Check sheet for the modelled part. Datum: model origin and axes. Units: mm. Face numbers are marked on the shaded views. A direction names the side the tool comes from. Give positions to 0.01 mm unless a question says otherwise; leave off trailing zeros. Write each loop counter-clockwise with the first axis right and the second up, starting at its lowest first coordinate (ties: lowest second). Pieces come first, ordered by that corner, then holes. Notation, with made-up numbers: M -7.5,29 L 39.5,29 A22 ccw 39.5,47 Z; hole C 0.5,64.25 d2. An arc over 180 degrees is marked long. Write each question's results on one line, items separated by ' | '. Start each with the question number.
from build123d import *

# Parameters (mm, degrees)
SKETCH1_W                                  = 47
SKETCH1_H                                  = 47
BOSS_EXTRUDE1_DEPTH                        = 32
SKETCH2_W                                  = 44
SKETCH2_H                                  = 44
CUT_EXTRUDE1_DEPTH                         = 26.1
SKETCH3_W                                  = 3.5
SKETCH3_H                                  = 3.5
BOSS_EXTRUDE2_DEPTH                        = 20.5
MIRROR1_AT_THE_SECOND_PLANE_COPY_1_SKETC_W = 3.5
MIRROR1_AT_THE_SECOND_PLANE_COPY_1_SKETC_H = 3.5
MIRROR1_AT_THE_SECOND_PLANE_COPY_1_DEPTH   = 20.5
CUT_EXTRUDE3_REACH                         = 63.524
SKETCH4_W                                  = 2
SKETCH4_H                                  = 20
LPATTERN1_COUNT                            = 7
LPATTERN1_PITCH                            = 4
BOSS_EXTRUDE4_START                        = -1.5
SKETCH8_W                                  = 26
SKETCH8_H                                  = 2
BOSS_EXTRUDE4_DEPTH                        = 1.5
LPATTERN2_COUNT                            = 5
LPATTERN2_PITCH                            = 4
SKETCH6_W                                  = 47
SKETCH6_H                                  = 47
SKETCH6_W_2                                = 44
SKETCH6_H_2                                = 44
BOSS_EXTRUDE5_DEPTH                        = 3
SKETCH7_R                                  = 5
CUT_EXTRUDE4_DEPTH                         = 10
SKETCH10_W                                 = 10
SKETCH10_H                                 = 5
CUT_EXTRUDE5_DEPTH                         = 62.524385409
SKETCH12_W                                 = 12.571328749
SKETCH12_H                                 = 5
CUT_EXTRUDE6_DEPTH                         = 10


with BuildPart() as part:
    # Sketch1 → Boss-Extrude1 (new body)
    with BuildSketch(Plane(origin=(0, 0, 0), x_dir=(1, 0, 0), z_dir=(0, 1, 0))):
        Rectangle(SKETCH1_W, SKETCH1_H)
    extrude(amount=BOSS_EXTRUDE1_DEPTH)

    # Sketch2 → Cut-Extrude1 (cut)
    with BuildSketch(Plane.XZ):
        Rectangle(SKETCH2_W, SKETCH2_H)
    extrude(amount=-CUT_EXTRUDE1_DEPTH, mode=Mode.SUBTRACT)

    # Sketch3 → Boss-Extrude2 (add)
    with BuildSketch(Plane.XZ.offset(-26.1)):
        with Locations((-20.25, 20.25)):
            Rectangle(SKETCH3_W, SKETCH3_H)
    boss_extrude2 = extrude(amount=BOSS_EXTRUDE2_DEPTH)

    # Mirror1: Boss-Extrude2 across plane
    add(boss_extrude2.mirror(Plane(origin=(0, 0, 0), x_dir=(0, 0, 1), z_dir=(1, 0, 0))))

    # Mirror1 at the second plane: Boss-Extrude2 across plane
    add(boss_extrude2.mirror(Plane.XY))

    # Mirror1 at the second plane copy 1 sketc → Mirror1 at the second plane copy 1 (add)
    with BuildSketch(Plane(origin=(0, 26.1, 0), x_dir=(-1, 0, 0), z_dir=(0, -1, 0))):
        with Locations((-20.25, 20.25)):
            Rectangle(MIRROR1_AT_THE_SECOND_PLANE_COPY_1_SKETC_W, MIRROR1_AT_THE_SECOND_PLANE_COPY_1_SKETC_H)
    extrude(amount=MIRROR1_AT_THE_SECOND_PLANE_COPY_1_DEPTH)

    # Sketch4 → Cut-Extrude3 (cut, up to next)
    with BuildSketch(Plane(origin=(0, 0, -23.5), x_dir=(-1, 0, 0), z_dir=(0, 0, -1)), mode=Mode.PRIVATE) as cut_extrude3_sk1:
        with Locations((-12, 13.157296847)):
            Rectangle(SKETCH4_W, SKETCH4_H)
    cut_extrude3_tool1 = extrude(cut_extrude3_sk1.sketch, amount=-CUT_EXTRUDE3_REACH, mode=Mode.PRIVATE) & part.part
    cut_extrude3 = cut_extrude3_tool1.solids().sort_by_distance((12, 13.157297, -23.5))[0]
    add(cut_extrude3, mode=Mode.SUBTRACT)

    # LPattern1: Cut-Extrude3 ×7
    with Locations(*[(-i * LPATTERN1_PITCH, 0, 0) for i in range(1, LPATTERN1_COUNT)]):
        add(cut_extrude3, mode=Mode.SUBTRACT)

    # Sketch8 → Boss-Extrude4 (add)
    with BuildSketch(Plane(origin=(0, 0, -23.5), x_dir=(-1, 0, 0), z_dir=(0, 0, -1)).offset(BOSS_EXTRUDE4_START)):
        with Locations((0, 20.157296847)):
            Rectangle(SKETCH8_W, SKETCH8_H)
    boss_extrude4 = extrude(amount=BOSS_EXTRUDE4_DEPTH)

    # LPattern2: Boss-Extrude4 ×5
    with Locations(*[(0, -i * LPATTERN2_PITCH, 0) for i in range(1, LPATTERN2_COUNT)]):
        add(boss_extrude4)

    # Sketch6 → Boss-Extrude5 (add)
    with BuildSketch(Plane.XZ):
        Rectangle(SKETCH6_W, SKETCH6_H)
        Rectangle(SKETCH6_W_2, SKETCH6_H_2, mode=Mode.SUBTRACT)
    extrude(amount=BOSS_EXTRUDE5_DEPTH)

    # Sketch7 → Cut-Extrude4 (cut)
    with BuildSketch(Plane(origin=(0, 32, 0), x_dir=(1, 0, 0), z_dir=(0, 1, 0))):
        with Locations(Location((0, 0, 0), (0, 0, 270))):
            Circle(SKETCH7_R)
    extrude(amount=-CUT_EXTRUDE4_DEPTH, mode=Mode.SUBTRACT)

    # Sketch10 → Cut-Extrude5 (cut, through all)
    with BuildSketch(Plane.ZY.offset(23.5)):
        with Locations((8.871811033, 3.1)):
            Rectangle(SKETCH10_W, SKETCH10_H)
    extrude(amount=-CUT_EXTRUDE5_DEPTH, mode=Mode.SUBTRACT)

    # Sketch12 → Cut-Extrude6 (cut)
    with BuildSketch(Plane.XY.offset(23.5)):
        with Locations((-10.783165608, 3.1)):
            Rectangle(SKETCH12_W, SKETCH12_H)
    extrude(amount=-CUT_EXTRUDE6_DEPTH, mode=Mode.SUBTRACT)


solid = part.part
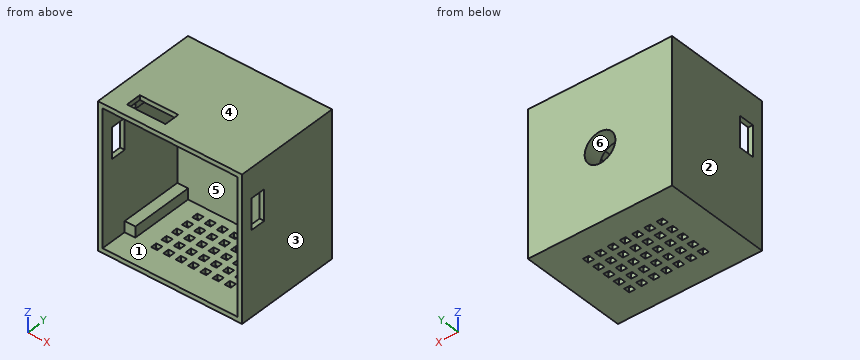
Q1. Scan lines: L1, parallel to X at y = 23.5, z = 20; L2, parallel to X at y = 28, z = 0; L3, parallel to Z at x = -6, y = 12.5. Record each from-to range of solid material in increasing order.
Q2. Section check C-C on x = 0. State how many separate pieces and enclosed holes the cut face has, plus the area to 3 significant figures.
Q3. Section check B-B on z = 0. Record the boundary of the cut face in (x, y), plus the area to 3 significant figures.
Q4. Tool access check on the marked faces 1 and 2. Record the directions out of +Z, -Z, +X, -X, +Y, -Y that give a thin tool (end or side, any length) a straight path to the whole face; none if there is none.
Q5. Release check for a two-part mould opening along X. For the marked faces 3, 4, 5 and 6 record: pulls with the +X half, pulls with the -X half, needs draft (parallel to the pull), parting line crosses it, or undercut.
Q6. Section check A-A on y = 16. Record the boundary of the cut face in (x, z).
Q7. Depth check by flat-ended pin: pin 1 Ø3 at (x, z) = (8, -2) entering from -Y. Enter the tip coordinate at first touch or a pass-through.
Check result:
1) L1: -23.5 to -18.5, 18.5 to 23.5 | L2: -23.5 to -5, 5 to 23.5 | L3: -23.5 to -22, 22 to 23.5
2) separate pieces: 7 | enclosed holes: 0 | area: 291 mm^2
3) outline: M -23.5,-3 L -22,-3 L -22,26.1 L -5,26.1 L -5,32 L -23.5,32 Z; M 5,26.1 L 22,26.1 L 22,-3 L 23.5,-3 L 23.5,32 L 5,32 Z | area: 306 mm^2
4) face 1: -Y | face 2: +Z, -Z, -X, +Y, -Y
5) face 3: pulls with the +X half | face 4: needs draft | face 5: undercut | face 6: undercut
6) outline: M -23.5,-23.5 L 23.5,-23.5 L 23.5,23.5 L -23.5,23.5 Z; hole M -22,-18.5 L -18.5,-18.5 L -18.5,-22 L 18.5,-22 L 18.5,-18.5 L 22,-18.5 L 22,18.5 L 18.5,18.5 L 18.5,22 L -18.5,22 L -18.5,18.5 L -22,18.5 Z
7) pin 1: y = 26.1
